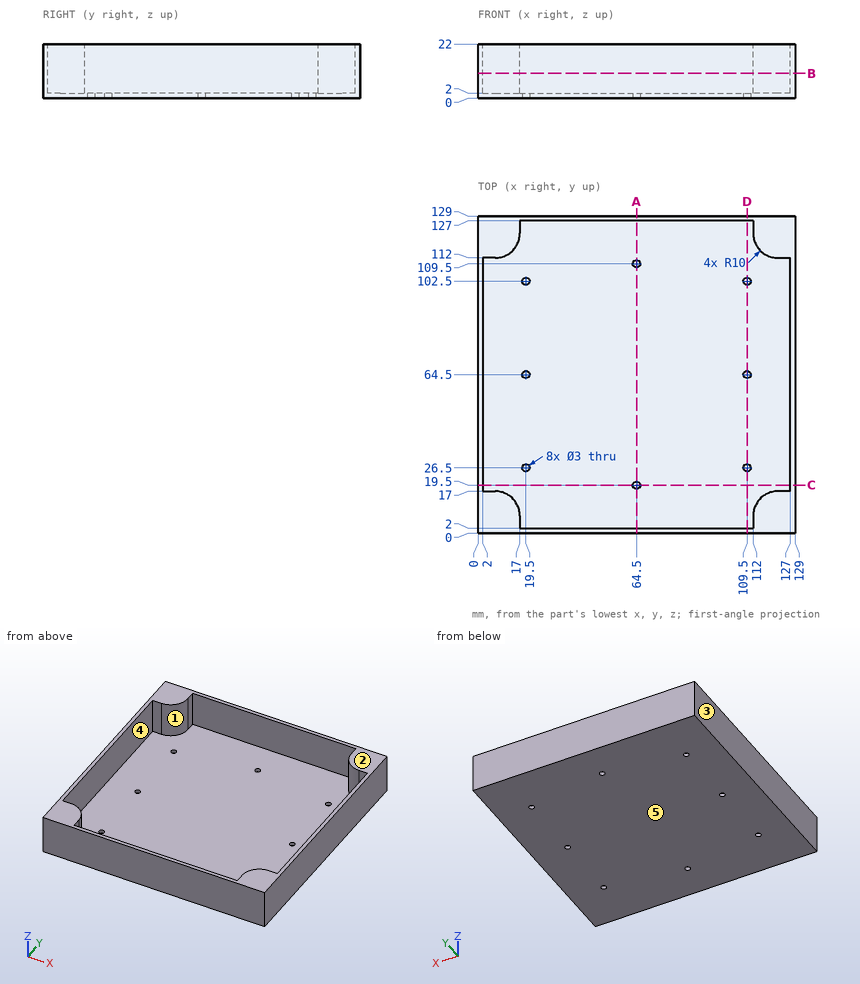
Here's the drawing with two shaded views (mm, measured from the low corner). I have some questions. A direction names the side the tool comes from. Coordinates: 2 decimals unless noted, no trailing zeros. Loops run counter-clockwise (first coordinate to the right, second up) from the corner with the lowest first, then second, coordinate; pieces in that order, holes last. Notation, with made-up numbers: (-23.5, 30) - (18.5, 30) arc R28 ccw to (18.5, 62) - close; hole circle Ø9 at (49, 57.5). An arc over 180 degrees is marked (long way). Answer as CSV lines item,"result". Start each with the question number.
1) Suppose I cut it at B-B (z = 10). Please give me the cut outline in (x, y), plus the area to 3 significant figures.
2) Suppose I cut it at C-C (y = 19.5). Please give me the cut outline in (x, z), plus the area to 3 significant figures.
3) For pin 1 (10 mm diameter, centred on x = 16.5, y = 102, fed in from +Z); pin 2 (2.5 mm diameter, centred on x = 109.5, y = 64.5, fed in from +Z), each with a flat end and sliding along its axis, tell me the tip position at first contact or that it passes through.
4) Which directions (+Z, -Z, +X, -X, +Y, -Y) give clear straight access to the entire face, cutting with the end or side of a thin tool? Please do the marked faces 1 and 2.
5) Thinking about a two-plate mould opening in X: for the marked faces 3, 4 and 5, which applies, pulls with the +X half, pulls with the -X half, needs draft (parallel to the pull), parting line crosses it, or undercut?
6) I need wall thicknesses on line 1 (X direction, y = 64.5, z = 1.55); line 2 (Y direction, x = 19.5, z = 1.5). Which ranges of each line are inside material? Lowest first, please. Write a range as from..to.
7) Suppose I cut it at D-D (x = 109.5). Please give me the cut outline in (y, z), plus the area to 3 significant figures.
8) Suppose I cut it at A-A (x = 64.5). Please give me the cut outline in (y, z).
Check result:
1,outline,"(0, 0) - (129, 0) - (129, 129) - (0, 129) - close; hole (2, 17) - (7, 17) arc R10 cw to (17, 7) - (17, 2) - (112, 2) - (112, 7) arc R10 cw to (122, 17) - (127, 17) - (127, 112) - (122, 112) arc R10 cw to (112, 122) - (112, 127) - (17, 127) - (17, 122) arc R10 cw to (7, 112) - (2, 112) - close"
1,area,"1,830 mm²"
2,outline,"(0, 0) - (63, 0) - (63, 2) - (2, 2) - (2, 22) - (0, 22) - close; (66, 0) - (129, 0) - (129, 22) - (127, 22) - (127, 2) - (66, 2) - close"
2,area,"332 mm²"
3,pin 1,"stops at z = 2"
3,pin 2,"passes through"
4,face 1,"+Z"
4,face 2,"+Z, +X, -X, +Y, -Y"
5,face 3,"pulls with the -X half"
5,face 4,"undercut"
5,face 5,"needs draft"
6,line 1,"x = 0..18, 21..108, 111..129"
6,line 2,"y = 0..25, 28..63, 66..101, 104..129"
7,outline,"(0, 0) - (25, 0) - (25, 2) - (2, 2) - (2, 22) - (0, 22) - close; (28, 0) - (63, 0) - (63, 2) - (28, 2) - close; (66, 0) - (101, 0) - (101, 2) - (66, 2) - close; (104, 0) - (129, 0) - (129, 22) - (127, 22) - (127, 2) - (104, 2) - close"
7,area,"320 mm²"
8,outline,"(0, 0) - (18, 0) - (18, 2) - (2, 2) - (2, 22) - (0, 22) - close; (21, 0) - (108, 0) - (108, 2) - (21, 2) - close; (111, 0) - (129, 0) - (129, 22) - (127, 22) - (127, 2) - (111, 2) - close"
